For this review, use the dimensioned drawing (mm, ordinates from the lowest corner) and the shaded views. A direction names the side the tool comes from. Round coordinates to 2 decimals unless told otherwise and drop trailing zeros. Order: outer loops, then holes, each group sorted by start corner. A loop starts at its lowest first (then second) coordinate and runs counter-clockwise, first axis right, second up. Notation, with made-up numbers: M 30,-25.5 L 65,-25.5 A30 cw 65,8.5 Z; hole C 40,20 d9. An arc over 180 degrees is marked long. Use a Markdown table: item, result. Add a question column.
1. To check wall thickness, follow probe 1 along X at (y, z) = (3.5, 1.65) (3 decimals); probe 2 along X at (y, z) = (3.5, 0.95); probe 3 along Y at (x, z) = (3.75, 0.8). State the ranges of each line that lie inside material, in increasing order.
2. For the marked faces 4, 5, 6 and 7, list the 3-axis set-ups (+Z, -Z, +X, -X, +Y, -Y) from which the entire face can be reached by the end or side of a thin tool; tool diameter is ignored.
3. Insertion check: P1, Ø1.5, axis at x = 5, y = 6, coming from the -Z side. The pin has a flat end and moves straight along its axis. Give the tip position at first contact, or say it passes through.
4. The part is to be moulded in two halves that separate along X. For the marked faces 1, 2 and 3, say which applies: +X half, -X half, draft (parallel to the pull), parting line (faces both ways), or undercut.
5. Consider section A-A on z = 0.15. State the section outline as (x, y) points (3 decimals), then the cut area to 3 significant figures.
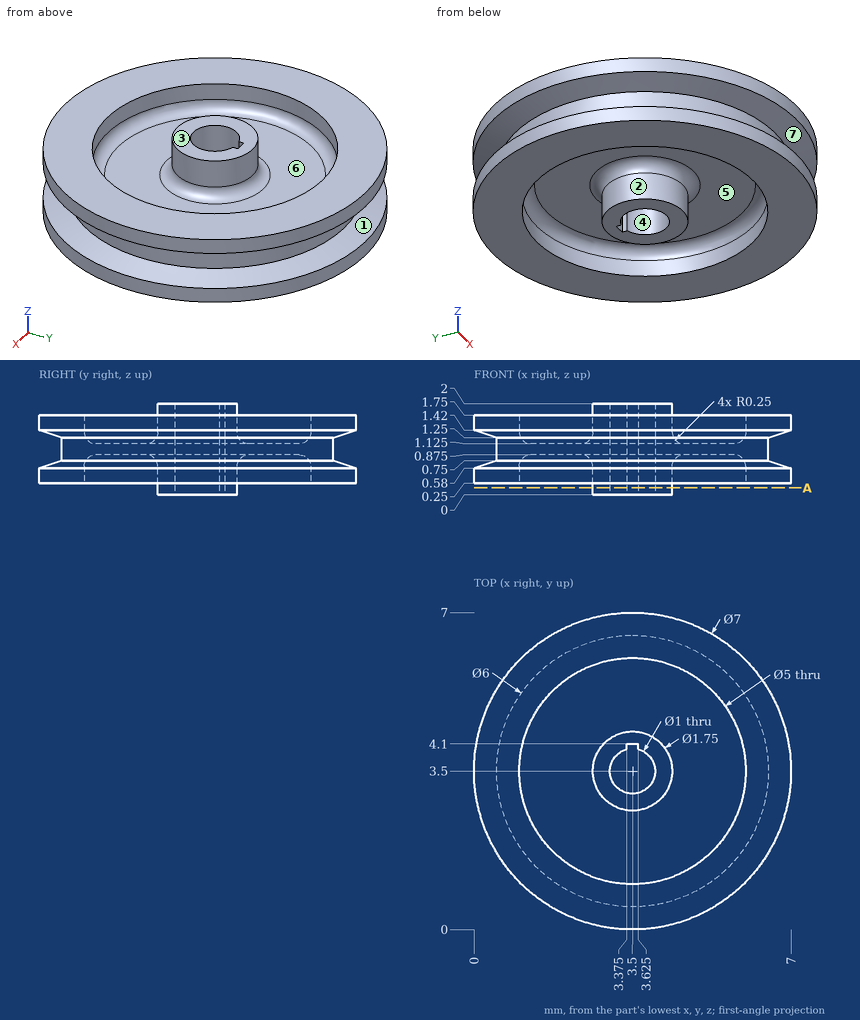
Answer block:
| question | item | result |
|---|---|---|
| 1 | probe 1 | 0 to 1, 2.625 to 3, 4 to 4.375, 6 to 7 |
| 1 | probe 2 | 0.5 to 3, 4 to 6.5 |
| 1 | probe 3 | 0.51 to 1.08, 2.59 to 3.07, 3.93 to 4.41, 5.92 to 6.49 |
| 2 | face 4 | +Z, -Z |
| 2 | face 5 | -Z |
| 2 | face 6 | +Z |
| 2 | face 7 | none |
| 3 | P1 | z = 0.25 |
| 4 | face 1 | parting line |
| 4 | face 2 | undercut |
| 4 | face 3 | draft |
| 5 | outline | C 3.5,3.5 d1.75; hole M 3.375,3.984 A0.5 ccw long 3.625,3.984 L 3.625,4.1 L 3.375,4.1 Z |
| 5 | area | 1.59 mm^2 |
